from build123d import *

# Parameters (mm, degrees)
FILLET1_R   = 0.2
HEX_2_DEPTH = 1.5


with BuildPart() as part:
    # BodySke → BaseBody (revolve)
    with BuildSketch(Plane.XY):
        with BuildLine():
            Line((12.75, 0), (12.75, 2.065))
            Line((12.75, 2.065), (12.315, 2.5))
            Line((12.315, 2.5), (2.75, 2.5))
            Line((2.75, 2.5), (2.75, 4.75))
            Line((2.75, 4.75), (2.37, 4.75))
            ThreePointArc((2.37, 4.75), (0.992680215, 3.754414901), (0, 2.375))
            Line((0, 2.375), (0, 0))
            Line((0, 0), (12.75, 0))
        make_face()
    revolve(axis=Axis((0, 0, 0), (1, 0, 0)))

    # Fillet1
    fillet1_edges = [part.edges().sort_by_distance(p)[0] for p in [
        (2.75, -2.5, 0),
    ]]
    fillet(fillet1_edges, radius=FILLET1_R)

    # Sketch2 → PreBroach (revolve, cut)
    with BuildSketch(Plane.XY):
        Polygon((0, 1.25), (1.3, 1.25), (2.021687836, 0), (0, 0), align=None)
    revolve(axis=Axis((0, 0, 0), (1, 0, 0)), mode=Mode.SUBTRACT)

    # Sketch3 → Hex 2 (cut)
    with BuildSketch(Plane(origin=(0, 0, 0), x_dir=(0, 0, -1), z_dir=(1, 0, 0))):
        Polygon((-1.5, -0.866025404), (-1.5, 0.866025404), (0, 1.732050808), (1.5, 0.866025404), (1.5, -0.866025404), (0, -1.732050808), align=None)
    extrude(amount=HEX_2_DEPTH, mode=Mode.SUBTRACT)


solid = part.part
The listing builds one solid part. Answer for the finished solid, in the listing's coordinates (mm). A direction names the side the tool comes from. Give positions to 0.01 mm unless a question says otherwise; leave off trailing zeros. Loops run counter-clockwise (first coordinate to the right, second up) from the corner with the lowest first, then second, coordinate; pieces in that order, holes last.
Item 1: A cutting plane is placed at B-B (y = 3). Give the vertices of the cut face in (x, z).
Derived:
outline: (2.37, -3.68) - (2.75, -3.68) - (2.75, 3.68) - (2.37, 3.68) arc R4.39 ccw to start
Item 2: Each of these flat-tipped pins is pushed along its axis until it touches: pin 1 Ø1.5 at (y, z) = (1.5, -3.5) entering from +X; pin 2 Ø4 at (x, z) = (9, -1.5) entering from +Y; pin 3 Ø0.8 at (x, y) = (0.5, -0.5) entering from -Z. Where does it stop, or does it pass through?
Derived:
pin 1: stops at x = 2.75
pin 2: stops at y = 2.5
pin 3: stops at z = -3.63
Item 3: A cutting plane is placed at A-A (x = 7.75). Give the vertices of the cut face in (y, z), then the cut area to 3 significant figures.
Derived:
outline: circle Ø5 at (0, 0)
area: 19.6 mm2
Item 4: A tool of negligible diameter and unlimited length cuts with its end or side. For faces 1 (the cylindrical face through (2.557, 2.192, -4.214)), 2 (the flat face through (2.75, -2.04, -2.04)), 3 (the flat face through (0.74, -1.293, -0.76)), from which of +Z, -Z, +X, -X, +Y, -Y can it reach the whole face along a straight path? Write none if from no direction.
Derived:
face 1: +X, -X
face 2: +X
face 3: -X
Item 5: Find the intervals of material crossed by line 1 along Z through (x, y) = (10.5, 2); line 2 along X through (y, z) = (0.75, 1.25); line 3 along X through (y, z) = (1.25, 4.5), in increasing order.
Derived:
line 1: z = -1.5 to 1.5
line 2: x = 1.5 to 12.75
line 3: x = 2.22 to 2.75
Item 6: Determine the mould class of faces 4 (the cylindrical face through (7.57, -0.54, -2.44)), 5 (the flat face through (0, 0, -2)), 6 (the flat face through (1, 0, 1.5)) for opening direction Z: +Z half, -Z half, draft (parallel to the pull), parting line (faces both ways), or undercut.
Derived:
face 4: parting line
face 5: draft
face 6: undercut
